Work out the finished part from the listing and answer in its coordinate system (mm). Give positions to 0.01 mm unless a question says otherwise; leave off trailing zeros. Order: outer loops, then holes, each group sorted by start corner. A loop starts at its lowest first (then second) coordinate and runs counter-clockwise, first axis right, second up. Notation, with made-up numbers: (27.25, 71) - (81.25, 71) arc R31 cw to (81.25, 105) - close; hole circle Ø8 at (59.5, -5.5). An arc over 180 degrees is marked (long way). Write each question's results on one line, items separated by ' | '.
Autodesk Inventor part; units mm, degrees
ref_plane "YZ Plane" through (0, 0, 0) normal (1, 0, 0) x (0, 1, 0)
ref_plane "XZ Plane" through (0, 0, 0) normal (0, 1, 0) x (-1, 0, 0)
ref_plane "XY Plane" through (0, 0, 0) normal (0, 0, 1) x (1, 0, 0)
sketch "Sketch1" plane through (0, 0, 0) normal (0, 1, 0) x (-1, 0, 0)
  circle A0 centre (0, 0) radius 138.938
  dimension "d0" = 277.876
extrude "Extrusion1" add sketch "Sketch1" along normal blind 25.4
fillet "Fillet1" radius 25.4 1 edges at (138.938, 25.4, 0)
shell "Shell1" thickness 2.54 removed faces 2 at (78.7519, 0.0001, -114.4636) at (28.4576, 0, -60.367)
properties part number "Frisbee" material "Glass"
1. A cutting plane is placed at A-A, the plane y = 7.75. Write down the section's boundary in (x, z).
Answer list:
outline: circle Ø275.45 at (0, 0); hole circle Ø270.09 at (0, 0)
2. Straight lines are drawn through the part: line 1 (Y direction, x = 61, z = -80.5); line 2 (X direction, y = 11.5, z = -11.5); line 3 (X direction, y = 11, z = 122.5). For each, find the intervals that lie inside material, in ascending order. Write a range as [from, to].
Answer list:
line 1: [22.86, 25.4] | line 2: [-135.7, -132.8], [132.8, 135.7] | line 3: [-60.06, -53.26], [53.26, 60.06]
3. Determine the mould class of faces 1 (the face through (2, 22.86, 2)), 2 (the face through (-92, 0, -102)) for opening direction Z: +Z half, -Z half, draft (parallel to the pull), parting line (faces both ways), or undercut.
Answer list:
face 1: undercut | face 2: draft
4. Given P1, Ø4, axis at y = 20.5, z = 106.5, coming from the -X side; P2, Ø8, axis at y = 22.5, z = 35, coming from the +X side; P3, Ø2, axis at x = 72, y = 19, coming from the +Z side, each flat-ended and moving along its own axis, determine where each tip first touches the part or whether it passes through.
Answer list:
P1: x = -77.1 | P2: x = 126.31 | P3: z = 110.15
